```python
from build123d import *

# Parameters (mm, degrees)
SKETCH1_W           = 85
SKETCH1_H           = 105
BOSS_EXTRUDE1_DEPTH = 17
SHELL1_T            = -2
SKETCH3_W           = 13
SKETCH3_H           = 6
CUT_EXTRUDE1_DEPTH  = 10
FILLET1_R           = 5


with BuildPart() as part:
    # Sketch1 → Boss-Extrude1 (new body)
    with BuildSketch(Plane(origin=(0, 0, 0), x_dir=(1, 0, 0), z_dir=(0, 1, 0))):
        Rectangle(SKETCH1_W, SKETCH1_H)
    extrude(amount=BOSS_EXTRUDE1_DEPTH)

    # Shell1
    shell1_openings = [part.faces().sort_by_distance(p)[0] for p in [
        (0, 17, 0),
    ]]
    offset(amount=SHELL1_T, openings=shell1_openings, kind=Kind.INTERSECTION)

    # Sketch3 → Cut-Extrude1 (cut)
    with BuildSketch(Plane(origin=(42.5, 0, 0), x_dir=(0, 0, -1), z_dir=(1, 0, 0))):
        with Locations((-4, 13)):
            Rectangle(SKETCH3_W, SKETCH3_H)
    extrude(amount=-CUT_EXTRUDE1_DEPTH, mode=Mode.SUBTRACT)

    # Fillet1
    fillet1_edges = [part.edges().sort_by_distance(p)[0] for p in [
        (42.5, 8.5, 52.5),
        (-42.5, 8.5, 52.5),
        (-42.5, 8.5, -52.5),
        (42.5, 8.5, -52.5),
    ]]
    fillet(fillet1_edges, radius=FILLET1_R)


solid = part.part
```
Could you check a few things on this model? Use its own coordinates, in mm. A direction names the side the tool comes from. Round coordinates to 2 decimals unless told otherwise and drop trailing zeros. Loops run counter-clockwise (first coordinate to the right, second up) from the corner with the lowest first, then second, coordinate; pieces in that order, holes last. Notation, with made-up numbers: (-15.5, 51.5) -> (33.5, 51.5) arc R17 ccw to (33.5, 64.5) -> close; hole circle Ø5 at (8.5, 79). An arc over 180 degrees is marked (long way). One line per question, with ' | ' between items.
(1) If we section it at B-B on x = -22: List the corners of the cut face in (y, z) for me, and give its area (3 significant figures).
Model answer:
outline: (0, -52.5) -> (17, -52.5) -> (17, -50.5) -> (2, -50.5) -> (2, 50.5) -> (17, 50.5) -> (17, 52.5) -> (0, 52.5) -> close | area: 270 mm^2
(2) If I drill on probe 1 along Z at (x, y) = (-2, 13.5); probe 2 along X at (y, z) = (5.5, -28); probe 3 along Y at (x, z) = (4.5, 17), over which ranges is the centre line in solid material (lowest first)?
Model answer:
probe 1: z = -52.5 to -50.5, 50.5 to 52.5 | probe 2: x = -42.5 to -40.5, 40.5 to 42.5 | probe 3: y = 0 to 2
(3) For faces 1 (the face through (-40.5, 9, 1)), 2 (the face through (41, 8.62, 51.07)), which set-ups out of +Z, -Z, +X, -X, +Y, -Y let a thin tool reach every point of the face, with its end or its side?
Model answer:
face 1: +Y | face 2: +Z, +X, +Y, -Y
(4) If we section it at A-A on y = 8.5: List the corners of the cut face in (x, z) for me, and give its area (3 significant figures).
Model answer:
outline: (-42.5, -47.5) arc R5 ccw to (-37.5, -52.5) -> (37.5, -52.5) arc R5 ccw to (42.5, -47.5) -> (42.5, 47.5) arc R5 ccw to (37.5, 52.5) -> (-37.5, 52.5) arc R5 ccw to (-42.5, 47.5) -> close; hole (-40.5, -50.5) -> (40.5, -50.5) -> (40.5, 50.5) -> (-40.5, 50.5) -> close | area: 723 mm^2
(5) For pin 1 Ø0.6 at (x, y) = (42, 12.5) entering from +Z; pin 2 Ø1.6 at (x, y) = (41.5, 13) entering from -Z; pin 3 Ø10 at (x, z) = (21, 23.5) entering from +Y, each with a flat end and sliding along its axis, tell me the tip position at first contact or that it passes through.
Model answer:
pin 1: stops at z = 50.21 | pin 2: stops at z = -51.34 | pin 3: stops at y = 2
(6) Thinking about a two-plate mould opening in X: for faces 3 (the face through (-1, 8, 52.5)), 4 (the face through (-1, 9, -50.5)), 5 (the face through (41, 8.62, -51.07)), 6 (the face through (-1, 2, -1)), which applies, released by +X, released by -X, zero draft, split by the parting line, or undercut?
Model answer:
face 3: zero draft | face 4: undercut | face 5: released by +X | face 6: undercut
(7) If we section it at C-C on z = 25.5: List the corners of the cut face in (x, y) for me, and give its area (3 significant figures).
Model answer:
outline: (-42.5, 0) -> (42.5, 0) -> (42.5, 17) -> (40.5, 17) -> (40.5, 2) -> (-40.5, 2) -> (-40.5, 17) -> (-42.5, 17) -> close | area: 230 mm^2
